```python
from build123d import *

# Parameters (mm, degrees)
SKETCH5_R           = 4
BOSS_EXTRUDE2_DEPTH = 10
SKETCH6_R           = 2.75
CUT_EXTRUDE4_DEPTH  = 5.2
SKETCH7_R           = 2.2
CUT_EXTRUDE5_DEPTH  = 1
SKETCH9_R           = 1.35
CUT_EXTRUDE6_DEPTH  = 15.623631801
SKETCH10_R          = 1.35
CUT_EXTRUDE7_DEPTH  = 16.81440762
SKETCH11_R          = 1.35
CUT_EXTRUDE8_DEPTH  = 17.02035176


with BuildPart() as part:
    # Sketch5 → Boss-Extrude2 (new body)
    with BuildSketch(Plane.XY):
        with Locations((7.579960637, 0)):
            Circle(SKETCH5_R)
    extrude(amount=BOSS_EXTRUDE2_DEPTH)

    # Sketch6 → Cut-Extrude4 (cut)
    with BuildSketch(Plane(origin=(0, 0, 0), x_dir=(-1, 0, 0), z_dir=(0, 0, -1))):
        with Locations((-7.579960637, 0)):
            Circle(SKETCH6_R)
    extrude(amount=-CUT_EXTRUDE4_DEPTH, mode=Mode.SUBTRACT)

    # Sketch7 → Cut-Extrude5 (cut)
    with BuildSketch(Plane(origin=(0, 0, 5.2), x_dir=(-1, 0, 0), z_dir=(0, 0, -1))):
        with Locations((-7.579960637, 0)):
            Circle(SKETCH7_R)
    extrude(amount=-CUT_EXTRUDE5_DEPTH, mode=Mode.SUBTRACT)

    # Sketch9 → Cut-Extrude6 (cut, through all)
    with BuildSketch(Plane(origin=(-0.808601663, 0.683388857, 6.2), x_dir=(-1, 0, 0), z_dir=(0, 0, -1))):
        with Locations((-8.28220496, 0.932237564)):
            Circle(SKETCH9_R)
    extrude(amount=-CUT_EXTRUDE6_DEPTH, mode=Mode.SUBTRACT)

    # Sketch10 → Cut-Extrude7 (cut, through all)
    with BuildSketch(Plane.XY.offset(10)):
        with Locations((6.079595945, -1.307435574)):
            Circle(SKETCH10_R)
    extrude(amount=-CUT_EXTRUDE7_DEPTH, mode=Mode.SUBTRACT)

    # Sketch11 → Cut-Extrude8 (cut, through all)
    with BuildSketch(Plane(origin=(0, 0.749334917, 10), x_dir=(1, 0, 0), z_dir=(0, 0, 1))):
        with Locations((9.207532027, -2.067387295)):
            Circle(SKETCH11_R)
    extrude(amount=-CUT_EXTRUDE8_DEPTH, mode=Mode.SUBTRACT)


solid = part.part
```
Input: part model. Units: mm. Frame: model coordinates. A direction names the side the tool comes from. Round coordinates to 2 decimals unless told otherwise and drop trailing zeros. Write each loop counter-clockwise with the first axis right and the second up, starting at its lowest first coordinate (ties: lowest second). Pieces come first, ordered by that corner, then holes. Notation, with made-up numbers: (23.5, -2) -> (53.5, -2) arc R6 cw to (53.5, 8) -> close; hole circle Ø1 at (76.25, 63). An arc over 180 degrees is marked (long way). Answer as CSV lines item,"result".
1. Ray query, L1, parallel to Y at x = 6.75, z = 9.5; L2, parallel to X at y = -2.25, z = 5.25; L3, parallel to X at y = -0.25, z = 6.75. Return the intervals inside material, ascending. Write a range as [from, to].
Geometry says:
L1,"y = [-3.91, -2.48], [-0.14, 0.48], [2.76, 3.91]"
L2,"x = [4.27, 5.11], [7.05, 8.23], [10.18, 10.89]"
L3,"x = [3.59, 5.24], [6.92, 8.38], [10.03, 11.57]"
2. Contact query for flat-ended pins moving along their axis: P1, Ø2.5, axis at x = 8.5, y = 0.5, coming from the -Z side; P2, Ø3, axis at y = 3, z = 8.5, coming from the +X side; P3, Ø2, axis at x = 7.47, y = 1.62, coming from the +Z side. Output: stop coordinate, or through.
Geometry says:
P1,"stops at z = 5.2"
P2,"stops at x = 11.29"
P3,"stops at z = 6.2"
3. Reachability of faces 1 (the flat face through (7, 3, 0)), 2 (the cylindrical face through (7.6, -2.2, 5.7)), 3 (the flat face through (7.5, 2.5, 6.2)) from +Z, -Z, +X, -X, +Y, -Y: full face, straight path, thin tool, end or side. Return the list, or none.
Geometry says:
face 1,"-Z, +X, -X, +Y, -Y"
face 2,"-Z"
face 3,"+Z"
4. Section C-C (z = 5.75). Return the cut outline in (x, y), plus the area to 3 significant figures.
Geometry says:
outline,"circle Ø8 at (7.58, 0); hole (5.39, -0.15) arc R1.35 ccw (long way) to (7.13, -2.15) arc R2.2 ccw to (8.13, -2.13) arc R1.35 ccw (long way) to (9.78, -0.09) arc R2.2 ccw (long way) to start"
area,"29.4 mm^2"
5. Mould query, pull axis X, two halves, no side actions, for faces 4 (the cylindrical face through (4.406, -2.434, 4.93)), 5 (the flat face through (8, 0, 10)), 6 (the cylindrical face through (5.01, -2.13, 6.18)). Classes: +X half, -X half, draft (parallel to the pull), parting line (faces both ways), or undercut.
Geometry says:
face 4,"parting line"
face 5,"draft"
face 6,"undercut"
6. Section D-D (x = 9.5). Return the cut outline in (y, z).
Geometry says:
outline,"(-3.51, 0) -> (-2.64, 0) -> (-2.64, 10) -> (-3.51, 10) -> close; (0, 6.2) -> (1.07, 6.2) -> (1.07, 5.2) -> (1.97, 5.2) -> (1.97, 0) -> (3.51, 0) -> (3.51, 10) -> (0, 10) -> close"
7. Section B-B (y = 1). Return the cut outline in (x, z), plus the area to 3 significant figures.
Geometry says:
outline,"(3.71, 0) -> (5.02, 0) -> (5.02, 5.2) -> (5.62, 5.2) -> (5.62, 6.2) -> (6.27, 6.2) -> (6.27, 10) -> (3.71, 10) -> close; (8.68, 6.2) -> (9.54, 6.2) -> (9.54, 5.2) -> (10.14, 5.2) -> (10.14, 0) -> (11.45, 0) -> (11.45, 10) -> (8.68, 10) -> close"
area,"37.8 mm^2"
8. Section A-A (x = 7). Return the cut outline in (y, z).
Geometry says:
outline,"(-3.96, 0) -> (-2.69, 0) -> (-2.69, 5.2) -> (-2.3, 5.2) -> (-2.3, 10) -> (-3.96, 10) -> close; (-0.32, 6.2) -> (0.35, 6.2) -> (0.35, 10) -> (-0.32, 10) -> close; (2.12, 5.2) -> (2.69, 5.2) -> (2.69, 0) -> (3.96, 0) -> (3.96, 10) -> (2.88, 10) -> (2.88, 6.2) -> (2.12, 6.2) -> close"
